```python
from build123d import *
from build123d.topology import SkipClean

# Parameters (mm, degrees)
SKETCH2_R           = 14.2875
SKETCH2_R_2         = 2.4892
SKETCH2_R_3         = 10.795
SKETCH2_R_4         = 1.778
BOSS_EXTRUDE1_DEPTH = 3.175
FILLET1_R           = 7.62
BOSS_EXTRUDE2_START = 2.38125
SKETCH4_R           = 14.2875
SKETCH4_R_2         = 1.778
SKETCH4_R_3         = 10.795
SKETCH4_R_4         = 2.4892
BOSS_EXTRUDE2_DEPTH = 2.38125


with BuildPart() as part:
    # Sketch2 → Boss-Extrude1 (new body)
    with BuildSketch(Plane.XY):
        with BuildLine():
            Line((142.632381685, 122.462939957), (142.632381685, -29.937060043))
            Line((142.632381685, -29.937060043), (142.632381685, -56.741928905))
            Line((142.632381685, -56.741928905), (142.632381685, -62.620500771))
            ThreePointArc((142.632381685, -62.620500771), (141.144484133, -66.21260322), (137.552381685, -67.700500771))
            Line((137.552381685, -67.700500771), (-137.552381685, -67.700500771))
            ThreePointArc((-137.552381685, -67.700500771), (-141.144484133, -66.21260322), (-142.632381685, -62.620500771))
            Line((-142.632381685, -62.620500771), (-142.632381685, -56.741928905))
            Line((-142.632381685, -56.741928905), (-142.632381685, -29.937060043))
            Line((-142.632381685, -29.937060043), (-142.632381685, 122.462939957))
            ThreePointArc((-142.632381685, 122.462939957), (-134.600001748, 148.101160684), (-108.918256202, 140.209048469))
            Line((-108.918256202, 140.209048469), (-31.75, 0))
            ThreePointArc((-31.75, 0), (0, -31.75), (31.75, 0))
            Line((31.75, 0), (108.918256202, 140.209048469))
            ThreePointArc((108.918256202, 140.209048469), (134.600001748, 148.101160684), (142.632381685, 122.462939957))
        make_face()
        with Locations((-60.484532313, 12.7)):
            Circle(SKETCH2_R, mode=Mode.SUBTRACT)
        with Locations((-125.726814921, 131.243846084)):
            Circle(SKETCH2_R, mode=Mode.SUBTRACT)
        with Locations((125.726814921, 131.243846084)):
            Circle(SKETCH2_R, mode=Mode.SUBTRACT)
        with Locations((60.484532313, 12.7)):
            Circle(SKETCH2_R, mode=Mode.SUBTRACT)
        with Locations((-76.5175, -57.15)):
            Circle(SKETCH2_R_2, mode=Mode.SUBTRACT)
        with Locations((-63.8175, -57.15)):
            Circle(SKETCH2_R_2, mode=Mode.SUBTRACT)
        with Locations((-51.1175, -57.15)):
            Circle(SKETCH2_R_2, mode=Mode.SUBTRACT)
        with Locations((-38.4175, -57.15)):
            Circle(SKETCH2_R_2, mode=Mode.SUBTRACT)
        with Locations((-25.7175, -57.15)):
            Circle(SKETCH2_R_2, mode=Mode.SUBTRACT)
        with Locations((-13.0175, -57.15)):
            Circle(SKETCH2_R_2, mode=Mode.SUBTRACT)
        with Locations((-0.3175, -57.15)):
            Circle(SKETCH2_R_2, mode=Mode.SUBTRACT)
        with Locations((12.3825, -57.15)):
            Circle(SKETCH2_R_2, mode=Mode.SUBTRACT)
        with Locations((25.0825, -57.15)):
            Circle(SKETCH2_R_2, mode=Mode.SUBTRACT)
        with Locations((37.7825, -57.15)):
            Circle(SKETCH2_R_2, mode=Mode.SUBTRACT)
        with Locations((50.4825, -57.15)):
            Circle(SKETCH2_R_2, mode=Mode.SUBTRACT)
        with Locations((63.1825, -57.15)):
            Circle(SKETCH2_R_2, mode=Mode.SUBTRACT)
        with Locations((75.8825, -57.15)):
            Circle(SKETCH2_R_2, mode=Mode.SUBTRACT)
        with Locations((-117.232381685, -16.900500771)):
            Circle(SKETCH2_R_3, mode=Mode.SUBTRACT)
        with Locations((117.232381685, -16.900500771)):
            Circle(SKETCH2_R_3, mode=Mode.SUBTRACT)
        with Locations((-135.647381685, -16.900500771)):
            Circle(SKETCH2_R_4, mode=Mode.SUBTRACT)
        with Locations((-126.439881685, -0.95264296)):
            Circle(SKETCH2_R_4, mode=Mode.SUBTRACT)
        with Locations((-108.024881685, -0.95264296)):
            Circle(SKETCH2_R_4, mode=Mode.SUBTRACT)
        with Locations((-98.817381685, -16.900500771)):
            Circle(SKETCH2_R_4, mode=Mode.SUBTRACT)
        with Locations((-108.024881685, -32.848358582)):
            Circle(SKETCH2_R_4, mode=Mode.SUBTRACT)
        with Locations((-126.439881685, -32.848358582)):
            Circle(SKETCH2_R_4, mode=Mode.SUBTRACT)
        with Locations((99.452381685, -16.900500771)):
            Circle(SKETCH2_R_4, mode=Mode.SUBTRACT)
        with Locations((108.342381685, -1.502569092)):
            Circle(SKETCH2_R_4, mode=Mode.SUBTRACT)
        with Locations((126.122381685, -1.502569092)):
            Circle(SKETCH2_R_4, mode=Mode.SUBTRACT)
        with Locations((135.012381685, -16.900500771)):
            Circle(SKETCH2_R_4, mode=Mode.SUBTRACT)
        with Locations((126.122381685, -32.29843245)):
            Circle(SKETCH2_R_4, mode=Mode.SUBTRACT)
        with Locations((108.342381685, -32.29843245)):
            Circle(SKETCH2_R_4, mode=Mode.SUBTRACT)
    extrude(amount=BOSS_EXTRUDE1_DEPTH)

    # Fillet1
    fillet1_edges = [part.edges().sort_by_distance(p)[0] for p in [
        (-31.75, 0, 1.5875),
        (31.75, 0, 1.5875),
    ]]
    fillet(fillet1_edges, radius=FILLET1_R)

    # Sketch4 → Boss-Extrude2 (add)
    with SkipClean():  # the faces are left unmerged after this step: merging them gives an invalid solid
        with BuildSketch(Plane(origin=(0, 0, 0), x_dir=(-1, 0, 0), z_dir=(0, 0, -1)).offset(BOSS_EXTRUDE2_START)):
            with BuildLine():
                Line((-32.640582486, 1.618122906), (-108.918256202, 140.209048469))
                ThreePointArc((-108.918256202, 140.209048469), (-134.600001748, 148.101160684), (-142.632381685, 122.462939957))
                Line((-142.632381685, 122.462939957), (-142.632381685, -62.620500771))
                ThreePointArc((-142.632381685, -62.620500771), (-141.144484133, -66.21260322), (-137.552381685, -67.700500771))
                Line((-137.552381685, -67.700500771), (137.552381685, -67.700500771))
                ThreePointArc((137.552381685, -67.700500771), (141.144484133, -66.21260322), (142.632381685, -62.620500771))
                Line((142.632381685, -62.620500771), (142.632381685, 122.462939957))
                ThreePointArc((142.632381685, 122.462939957), (134.600001748, 148.101160684), (108.918256202, 140.209048469))
                Line((108.918256202, 140.209048469), (32.640582486, 1.618122906))
                ThreePointArc((32.640582486, 1.618122906), (31.988191315, 0.032870886), (31.706674385, -1.65810115))
                ThreePointArc((31.706674385, -1.65810115), (0, -31.75), (-31.706674385, -1.65810115))
                ThreePointArc((-31.706674385, -1.65810115), (-31.988191315, 0.032870886), (-32.640582486, 1.618122906))
            make_face()
            with Locations((125.726814921, 131.243846084)):
                Circle(SKETCH4_R, mode=Mode.SUBTRACT)
            with Locations((108.024881685, -32.848358582)):
                Circle(SKETCH4_R_2, mode=Mode.SUBTRACT)
            with Locations((126.439881685, -32.848358582)):
                Circle(SKETCH4_R_2, mode=Mode.SUBTRACT)
            with Locations((135.647381685, -16.900500771)):
                Circle(SKETCH4_R_2, mode=Mode.SUBTRACT)
            with Locations((126.439881685, -0.95264296)):
                Circle(SKETCH4_R_2, mode=Mode.SUBTRACT)
            with Locations((108.024881685, -0.95264296)):
                Circle(SKETCH4_R_2, mode=Mode.SUBTRACT)
            with Locations((98.817381685, -16.900500771)):
                Circle(SKETCH4_R_2, mode=Mode.SUBTRACT)
            with Locations((117.232381685, -16.900500771)):
                Circle(SKETCH4_R_3, mode=Mode.SUBTRACT)
            with Locations((60.484532313, 12.7)):
                Circle(SKETCH4_R, mode=Mode.SUBTRACT)
            with Locations((76.5175, -57.15)):
                Circle(SKETCH4_R_4, mode=Mode.SUBTRACT)
            with Locations((63.8175, -57.15)):
                Circle(SKETCH4_R_4, mode=Mode.SUBTRACT)
            with Locations((51.1175, -57.15)):
                Circle(SKETCH4_R_4, mode=Mode.SUBTRACT)
            with Locations((38.4175, -57.15)):
                Circle(SKETCH4_R_4, mode=Mode.SUBTRACT)
            with Locations((25.7175, -57.15)):
                Circle(SKETCH4_R_4, mode=Mode.SUBTRACT)
            with Locations((13.0175, -57.15)):
                Circle(SKETCH4_R_4, mode=Mode.SUBTRACT)
            with Locations((0.3175, -57.15)):
                Circle(SKETCH4_R_4, mode=Mode.SUBTRACT)
            with Locations((-12.3825, -57.15)):
                Circle(SKETCH4_R_4, mode=Mode.SUBTRACT)
            with Locations((-25.0825, -57.15)):
                Circle(SKETCH4_R_4, mode=Mode.SUBTRACT)
            with Locations((-37.7825, -57.15)):
                Circle(SKETCH4_R_4, mode=Mode.SUBTRACT)
            with Locations((-50.4825, -57.15)):
                Circle(SKETCH4_R_4, mode=Mode.SUBTRACT)
            with Locations((-63.1825, -57.15)):
                Circle(SKETCH4_R_4, mode=Mode.SUBTRACT)
            with Locations((-75.8825, -57.15)):
                Circle(SKETCH4_R_4, mode=Mode.SUBTRACT)
            with Locations((-99.452381685, -16.900500771)):
                Circle(SKETCH4_R_2, mode=Mode.SUBTRACT)
            with Locations((-108.342381685, -32.29843245)):
                Circle(SKETCH4_R_2, mode=Mode.SUBTRACT)
            with Locations((-126.122381685, -32.29843245)):
                Circle(SKETCH4_R_2, mode=Mode.SUBTRACT)
            with Locations((-135.012381685, -16.900500771)):
                Circle(SKETCH4_R_2, mode=Mode.SUBTRACT)
            with Locations((-126.122381685, -1.502569092)):
                Circle(SKETCH4_R_2, mode=Mode.SUBTRACT)
            with Locations((-108.342381685, -1.502569092)):
                Circle(SKETCH4_R_2, mode=Mode.SUBTRACT)
            with Locations((-117.232381685, -16.900500771)):
                Circle(SKETCH4_R_3, mode=Mode.SUBTRACT)
            with Locations((-60.484532313, 12.7)):
                Circle(SKETCH4_R, mode=Mode.SUBTRACT)
            with Locations((-125.726814921, 131.243846084)):
                Circle(SKETCH4_R, mode=Mode.SUBTRACT)
        extrude(amount=-BOSS_EXTRUDE2_DEPTH)


solid = part.part
```
Model file for the job. Use its own axes, mm. A direction names the side the tool comes from. Round coordinates to 2 decimals unless told otherwise and drop trailing zeros. Write each loop counter-clockwise with the first axis right and the second up, starting at its lowest first coordinate (ties: lowest second). Pieces come first, ordered by that corner, then holes. Notation, with made-up numbers: (67.5, -30) - (109.5, -30) arc R9 cw to (109.5, -19) - close; hole circle Ø4 at (-16, -31.5). An arc over 180 degrees is marked (long way). Use CSV: the item, a comma, the result in double quotes. Start each with the question number.
Item 1: Tool access for faces 4 (the face through (-142.632, 29, 0)), 5 (the face through (34, -6, -2.381)): list every direction of +Z, -Z, +X, -X, +Y, -Y with a clear straight run to the whole face (end or side of a thin tool).
Item 2: Band-saw the part on D-D (y = -22.5). Write the cut outline in (x, z) (3 decimals), and give its area (3 significant figures).
Item 3: Drill centre lines: L1, parallel to X at y = -8, z = 0.6; L2, parallel to Y at x = 120.5, z = 2.8; L3, parallel to Y at x = -53, z = 0.5. Where is each one in solid material? Low to high. Write a range as [from, to].
Item 4: Two-plate mould, pull along X, no slides. Class faces 1 (the face through (142.632, 31, 0)), 2 (the face through (34, -6, 3.175)), 3 (the face through (134.23, 148.29, 0.36)): released by +X, released by -X, zero draft, split by the parting line, or undercut.
Item 5: Band-saw the part on C-C (y = 64.5). Write the cut outline in (x, z) (3 decimals), and give its area (3 significant figures).
Item 6: Band-saw the part on A-A (y = 12.7). Write the cut outline in (x, z) (3 decimals).
Item 7: Pin check, flat tips, straight feed: P1, Ø2, axis at x = -98.82, y = -16.9, coming from the +Z side; P2, Ø3, axis at y = 78, z = 2.5, coming from the +X side; P3, Ø3, axis at y = 19.5, z = 0.5, coming from the -X side. Stop position of each tip, or through.
Item 8: Band-saw the part on B-B (x = 69.5). Write the cut outline in (y, z) (1 decimal), and give its area (3 significant figures).
Checked values:
1,face 4,"+Z, -Z, -X, -Y"
1,face 5,"-Z, +X, -X, +Y, -Y"
2,outline,"(-142.632, -2.381) - (-126.462, -2.381) - (-126.462, 3.175) - (-142.632, 3.175) - close; (-108.003, -2.381) - (-22.401, -2.381) - (-22.401, 3.175) - (-108.003, 3.175) - close; (22.401, -2.381) - (108.003, -2.381) - (108.003, 3.175) - (22.401, 3.175) - close; (126.462, -2.381) - (142.632, -2.381) - (142.632, 3.175) - (126.462, 3.175) - close"
2,area,"1,130 mm²"
3,L1,"x = [-142.63, -123.34], [-111.12, -30.73], [30.73, 111.12], [123.34, 142.63]"
3,L2,"y = [-67.7, -27.19], [-6.61, 117.95], [144.54, 149.56]"
3,L3,"y = [-67.7, -58.78], [-55.52, 0.53], [24.87, 38.61]"
4,face 1,"released by +X"
4,face 2,"zero draft"
4,face 3,"undercut"
5,outline,"(-142.632, -2.381) - (-67.25, -2.381) - (-67.25, 3.175) - (-142.632, 3.175) - close; (67.25, -2.381) - (142.632, -2.381) - (142.632, 3.175) - (67.25, 3.175) - close"
5,area,"838 mm²"
6,outline,"(-142.632, -2.381) - (-74.772, -2.381) - (-74.772, 3.175) - (-142.632, 3.175) - close; (-46.197, -2.381) - (-38.74, -2.381) - (-38.74, 3.175) - (-46.197, 3.175) - close; (38.74, -2.381) - (46.197, -2.381) - (46.197, 3.175) - (38.74, 3.175) - close; (74.772, -2.381) - (142.632, -2.381) - (142.632, 3.175) - (74.772, 3.175) - close"
7,P1,"passes through"
7,P2,"stops at x = 142.63"
7,P3,"stops at x = -142.63"
8,outline,"(-67.7, -2.4) - (1.6, -2.4) - (1.6, 3.2) - (-67.7, 3.2) - close; (23.8, -2.4) - (68.6, -2.4) - (68.6, 3.2) - (23.8, 3.2) - close"
8,area,"634 mm²"
